```python
from build123d import *

# Parameters (mm, degrees)
SKETCH1_W            = 45
SKETCH1_H            = 40
BOSS_EXTRUDE1_DEPTH  = 1.57
SKETCH2_W            = 25.91
SKETCH2_H            = 2.41
BOSS_EXTRUDE2_DEPTH  = 8.51
SKETCH3_W            = 45
SKETCH3_H            = 40
BOSS_EXTRUDE3_DEPTH  = 1.57
SKETCH4_W            = 25.91
SKETCH4_H            = 2.41
BOSS_EXTRUDE4_DEPTH  = 8.51
SKETCH5_W            = 15
SKETCH5_H            = 14.5
BOSS_EXTRUDE5_DEPTH  = 5
FILLET1_R            = 2.5
FILLET1_OF_MIRROR1_R = 2.5
SKETCH6_W            = 8
SKETCH6_H            = 10.5
BOSS_EXTRUDE6_DEPTH  = 6.5
CUT_EXTRUDE1_REACH   = 37.381
SKETCH7_R            = 1.6
FILLET2_R            = 1.5
FILLET3_R            = 1.5


with BuildPart() as part:
    # Sketch1 → Boss-Extrude1 (new body)
    with BuildSketch(Plane(origin=(0, 0, 0), x_dir=(1, 0, 0), z_dir=(0, 1, 0))):
        Rectangle(SKETCH1_W, SKETCH1_H)
    extrude(amount=BOSS_EXTRUDE1_DEPTH)

    # Sketch2 → Boss-Extrude2 (add)
    with BuildSketch(Plane(origin=(0, 1.57, 0), x_dir=(1, 0, 0), z_dir=(0, 1, 0))):
        with Locations((9.035, 18.285)):
            Rectangle(SKETCH2_W, SKETCH2_H)
        with Locations((-0.435, -18.285)):
            Rectangle(SKETCH2_W, SKETCH2_H)
    extrude(amount=BOSS_EXTRUDE2_DEPTH)

    # Sketch3 → Boss-Extrude3 (add)
    with BuildSketch(Plane(origin=(0, 10.08, 0), x_dir=(1, 0, 0), z_dir=(0, 1, 0))):
        Rectangle(SKETCH3_W, SKETCH3_H)
    extrude(amount=BOSS_EXTRUDE3_DEPTH)

    # Sketch4 → Boss-Extrude4 (add)
    with BuildSketch(Plane(origin=(0, 11.65, 0), x_dir=(1, 0, 0), z_dir=(0, 1, 0))):
        with Locations((-0.435, -18.285)):
            Rectangle(SKETCH4_W, SKETCH4_H)
    extrude(amount=BOSS_EXTRUDE4_DEPTH)

    # Sketch5 → Boss-Extrude5 (add)
    with BuildSketch(Plane(origin=(0, 11.65, 0), x_dir=(1, 0, 0), z_dir=(0, 1, 0))):
        with Locations((-15, 0)):
            Rectangle(SKETCH5_W, SKETCH5_H)
    boss_extrude5 = extrude(amount=BOSS_EXTRUDE5_DEPTH)

    # Fillet1
    fillet1_edges = [part.edges().sort_by_distance(p)[0] for p in [
        (-15, 16.65, 7.25),
        (-15, 16.65, -7.25),
    ]]
    fillet(fillet1_edges, radius=FILLET1_R)

    # Mirror1: Boss-Extrude5 across plane
    add(boss_extrude5.mirror(Plane(origin=(0, 0, 0), x_dir=(0, 0, 1), z_dir=(1, 0, 0))))

    # Fillet1 of Mirror1
    fillet1_of_mirror1_edges = [part.edges().sort_by_distance(p)[0] for p in [
        (15, 16.65, 7.25),
        (15, 16.65, -7.25),
    ]]
    fillet(fillet1_of_mirror1_edges, radius=FILLET1_OF_MIRROR1_R)

    # Sketch6 → Boss-Extrude6 (add)
    with BuildSketch(Plane(origin=(0, 11.65, 0), x_dir=(1, 0, 0), z_dir=(0, 1, 0))):
        with Locations((0, -8.5)):
            Rectangle(SKETCH6_W, SKETCH6_H)
    extrude(amount=BOSS_EXTRUDE6_DEPTH)

    # Sketch7 → Cut-Extrude1 (cut, up to next)
    with BuildSketch(Plane(origin=(0, 1.57, 0), x_dir=(1, 0, 0), z_dir=(0, 1, 0)), mode=Mode.PRIVATE) as cut_extrude1_sk1:
        with Locations(Location((17.5, -15, 0), (0, 0, 270))):
            Circle(SKETCH7_R)
    cut_extrude1_tool1 = extrude(cut_extrude1_sk1.sketch, amount=-CUT_EXTRUDE1_REACH, mode=Mode.PRIVATE) & part.part
    # Sketch7 → Cut-Extrude1 (cut, up to next)
    with BuildSketch(Plane(origin=(0, 1.57, 0), x_dir=(1, 0, 0), z_dir=(0, 1, 0)), mode=Mode.PRIVATE) as cut_extrude1_sk2:
        with Locations(Location((-17.5, 15, 0), (0, 0, 270))):
            Circle(SKETCH7_R)
    cut_extrude1_tool2 = extrude(cut_extrude1_sk2.sketch, amount=-CUT_EXTRUDE1_REACH, mode=Mode.PRIVATE) & part.part
    add(cut_extrude1_tool1.solids().sort_by_distance((17.5, 1.57, 15))[0], mode=Mode.SUBTRACT)
    add(cut_extrude1_tool2.solids().sort_by_distance((-17.5, 1.57, -15))[0], mode=Mode.SUBTRACT)

    # Fillet2
    fillet2_edges = [part.edges().sort_by_distance(p)[0] for p in [
        (22.5, 0.785, 20),
        (-22.5, 0.785, 20),
        (-22.5, 0.785, -20),
        (22.5, 0.785, -20),
    ]]
    fillet(fillet2_edges, radius=FILLET2_R)

    # Fillet3
    fillet3_edges = [part.edges().sort_by_distance(p)[0] for p in [
        (22.5, 10.865, 20),
        (22.5, 10.865, -20),
        (-22.5, 10.865, -20),
        (-22.5, 10.865, 20),
    ]]
    fillet(fillet3_edges, radius=FILLET3_R)


solid = part.part
```
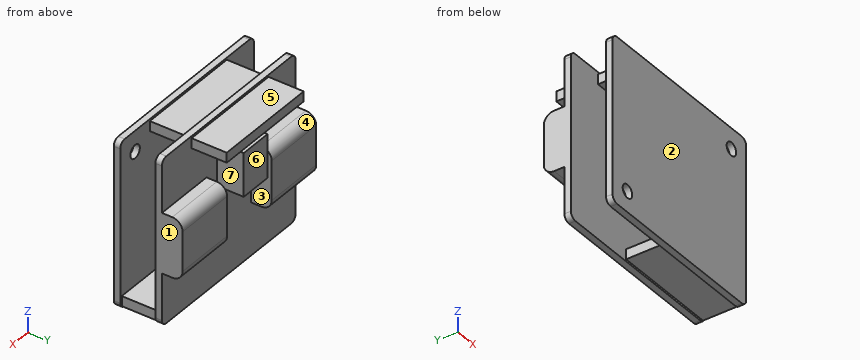
Geometry: final body of the model. Coordinates: model frame, mm. Face numbers are marked on the shaded views. A direction names the side the tool comes from. Round coordinates to 2 decimals unless told otherwise and drop trailing zeros. Write each loop counter-clockwise with the first axis right and the second up, starting at its lowest first coordinate (ties: lowest second). Pieces come first, ordered by that corner, then holes. Notation, with made-up numbers: M 17,33 L 76,33 A16 cw 76,48 Z; hole C 25.25,0.5 d8. An arc over 180 degrees is marked long. Answer in a Markdown table with one row per item. Add a question column.
(1) Ray query, L1, parallel to Y at x = -6, z = -7.5; L2, parallel to X at y = 0.4, z = -15; L3, parallel to Y at x = 17.5, z = -5. Return the intervals inside material, ascending.
(2) Draft query along X for the marked faces 1, 2 and 3. Return one class per face: pulls with the +X half, pulls with the -X half, needs draft (parallel to the pull), parting line crosses it, or undercut.
(3) Contact query for flat-ended pins moving along their axis: pin 1 (8 mm diameter, centred on x = 9, z = 7, fed in from +Y); pin 2 (2.5 mm diameter, centred on x = 0.5, z = 10.5, fed in from +Y); pin 3 (1.5 mm diameter, centred on x = 12, y = 8, fed in from -Z); pin 4 (3 mm diameter, centred on x = -5, y = 10, fed in from +Z). Output: stop coordinate, or through.
(4) Reachability of the marked faces 4, 5, 6 and 7 from +Z, -Z, +X, -X, +Y, -Y: full face, straight path, thin tool, end or side. Return the list, or none.
(5) Cut plane A-A, the plane y = 13.5. Return the cut outline in (x, z), then the cut area to 3 significant figures.
(6) Cut plane B-B, the plane y = 4.25. Return the cut outline in (x, z).
(7) Cut plane C-C, the plane x = 17.5. Return the cut outline in (y, z).
(8) Cut plane D-D, the plane z = -15. Return the cut outline in (x, y), then the cut area to 3 significant figures.
Established:
| question | item | result |
|---|---|---|
| 1 | L1 | 0 to 1.57, 10.08 to 11.65 |
| 1 | L2 | -22.5 to -19.1, -15.9 to 22.5 |
| 1 | L3 | 0 to 1.57, 10.08 to 16.64 |
| 2 | face 1 | pulls with the +X half |
| 2 | face 2 | needs draft |
| 2 | face 3 | undercut |
| 3 | pin 1 | y = 16.65 |
| 3 | pin 2 | y = 18.15 |
| 3 | pin 3 | z = -19.49 |
| 3 | pin 4 | z = 20 |
| 4 | face 4 | -X, +Y |
| 4 | face 5 | +Z, +X, -X, +Y |
| 4 | face 6 | -Z, +X, -X, +Y |
| 4 | face 7 | -Z, +Y |
| 5 | outline | M -22.5,-7.25 L -7.5,-7.25 L -7.5,7.25 L -22.5,7.25 Z; M -13.39,17.08 L 12.52,17.08 L 12.52,19.49 L -13.39,19.49 Z; M -4,3.25 L 4,3.25 L 4,13.75 L -4,13.75 Z; M 7.5,-7.25 L 22.5,-7.25 L 22.5,7.25 L 7.5,7.25 Z |
| 5 | area | 581 mm² |
| 6 | outline | M -13.39,17.08 L 12.52,17.08 L 12.52,19.49 L -13.39,19.49 Z; M -3.92,-19.49 L 21.99,-19.49 L 21.99,-17.08 L -3.92,-17.08 Z |
| 7 | outline | M 0,-20 L 1.57,-20 L 1.57,-19.49 L 10.08,-19.49 L 10.08,-20 L 11.65,-20 L 11.65,-7.25 L 14.15,-7.25 A2.5 ccw 16.65,-4.75 L 16.65,4.75 A2.5 ccw 14.15,7.25 L 11.65,7.25 L 11.65,20 L 10.08,20 L 10.08,-17.08 L 1.57,-17.08 L 1.57,13.4 L 0,13.4 Z; M 0,16.6 L 1.57,16.6 L 1.57,20 L 0,20 Z |
| 8 | outline | M -22.5,0 L -19.1,0 L -19.1,1.57 L -22.5,1.57 Z; M -22.5,10.08 L 22.5,10.08 L 22.5,11.65 L -22.5,11.65 Z; M -15.9,0 L 22.5,0 L 22.5,1.57 L -15.9,1.57 Z |
| 8 | area | 136 mm² |
